Read the model definition and answer for the solid it produces. Units are mm, in the model's axes. A direction names the side the tool comes from. Round coordinates to 2 decimals unless told otherwise and drop trailing zeros. Order: outer loops, then holes, each group sorted by start corner. A loop starts at its lowest first (then second) coordinate and runs counter-clockwise, first axis right, second up. Notation, with made-up numbers: (46.5, -40) - (82.5, -40) arc R23 cw to (82.5, -4) - close; hole circle Ø2 at (54.25, 17). An arc over 180 degrees is marked (long way). Answer as a JSON object with one key per item and string values. Group by question number.
Q1. A tool of negligible diameter and unlimited length cuts with its end or side. For faces 4 (the flat face through (2, 75, 110)), 5 (the flat face through (2.46, -9.75, -40.27)), 6 (the flat face through (2, -85, 100)), 7 (the cylindrical face through (2.465, -59.305, -21.258)), from which of +Z, -Z, +X, -X, +Y, -Y can it reach the whole face along a straight path? Write none if from no direction.
Q2. A cutting plane is placed at B-B on x = 1.5. Count the separate pieces of the cut face and the enclosed holes in it, and give its area (3 significant figures).
Q3. Given pin 1 Ø1 at (x, z) = (1, 12.5) entering from +Y; pin 2 Ø1 at (x, y) = (4, 36) entering from -Z; pin 3 Ø1.5 at (x, z) = (2.5, 103) entering from +Y, each flat-ended and moving along its own axis, determine where each tip first touches the part or whether it passes through.
Q4. Consider line 1 (Z direction, x = 3.6, y = 0); line 2 (Y direction, x = 1.5, z = -32.5); line 3 (Y direction, x = 0.65, z = -13). Determine where each line is inside the solid, lowest interval first.
Q5. The mould has two halves that part along Z. Classify faces 1 (the flat face through (2, 90, 102)), 2 (the cylindrical face through (2, -60, 3)), 3 (the flat face through (2, -75, 105)): pulls with the +Z half, pulls with the -Z half, needs draft (parallel to the pull), parting line crosses it, or undercut.
Q6. A cutting plane is placed at A-A on y = 0. Determine the outline of the cut face in (x, z).
```python
from build123d import *

# Parameters (mm, degrees)
F0_R     = 6.8
F3_DEPTH = 5
F4_DEPTH = 5.001
F5_DEPTH = 5


with BuildPart() as f3:
    # F0 (on Right) → F3 (new body)
    with BuildSketch(Plane.YZ):
        with BuildLine():
            ThreePointArc((15, -25.980762), (15.974572, -25.393169), (16.926158, -24.769037))
            add(Edge.make_bspline(
                [(16.926158, -24.769037), (45.375206, -5.328108), (94.536945, 53.480837), (100, 100)],
                knots=[0, 0, 0, 0, 149.895216, 149.895216, 149.895216, 149.895216], degree=3))
            Line((100, 100), (-90, 100))
            add(Edge.make_bspline(
                [(-33.810598, -54.161574), (-78.207154, -79.793938), (-84.736958, 0), (-90, 100)],
                knots=[0, 0, 0, 0, 164.082418, 164.082418, 164.082418, 164.082418], degree=3))
            Line((-33.810598, -54.161574), (15, -25.980762))
        make_face()
        Circle(F0_R, mode=Mode.SUBTRACT)
    extrude(amount=F3_DEPTH)

    # F1 (on Right) → F4 (cut, through all)
    with BuildSketch(Plane.YZ):
        with BuildLine():
            ThreePointArc((-57, 0), (-60, 3), (-63, 0))
            ThreePointArc((-63, 0), (-59.200635, -21.547269), (-48.2608, -40.495619))
            ThreePointArc((-48.2608, -40.495619), (-44.034304, -40.86539), (-43.664533, -36.638894))
            ThreePointArc((-43.664533, -36.638894), (-53.562479, -19.495148), (-57, 0))
        make_face()
    extrude(amount=F4_DEPTH, mode=Mode.SUBTRACT)

    # F2 (on Right) → F5 (join)
    with BuildSketch(Plane.YZ):
        Polygon((-80, 105), (-80, 100), (90, 100), (90, 105), (80, 105), (80, 110), (70, 110), (70, 115), (60, 115), (-50, 115), (-60, 115), (-60, 110), (-70, 110), (-70, 105), align=None)
    extrude(amount=F5_DEPTH)


solid = f3.part
```
Result set:
{
 "1": {"face 4": "+Z, +X, -X, +Y", "face 5": "-Z, +X, -X, +Y", "face 6": "+Z, +X, -X, -Y", "face 7": "+X, -X"},
 "2": {"separate pieces": "1", "enclosed holes": "2", "area": "23,000 mm²"},
 "3": {"pin 1": "stops at y = 55.94", "pin 2": "stops at z = -9.24", "pin 3": "stops at y = 90"},
 "4": {"line 1": "z = -34.64 to -6.8, 6.8 to 115", "line 2": "y = -74.07 to -53.97, -46.83 to 3.71", "line 3": "y = -79.2 to -61.64, -55.5 to 31.5"},
 "5": {"face 1": "needs draft", "face 2": "undercut", "face 3": "pulls with the +Z half"},
 "6": {"outline": "(0, -34.64) - (5, -34.64) - (5, -6.8) - (0, -6.8) - close; (0, 6.8) - (5, 6.8) - (5, 115) - (0, 115) - close"}
}
